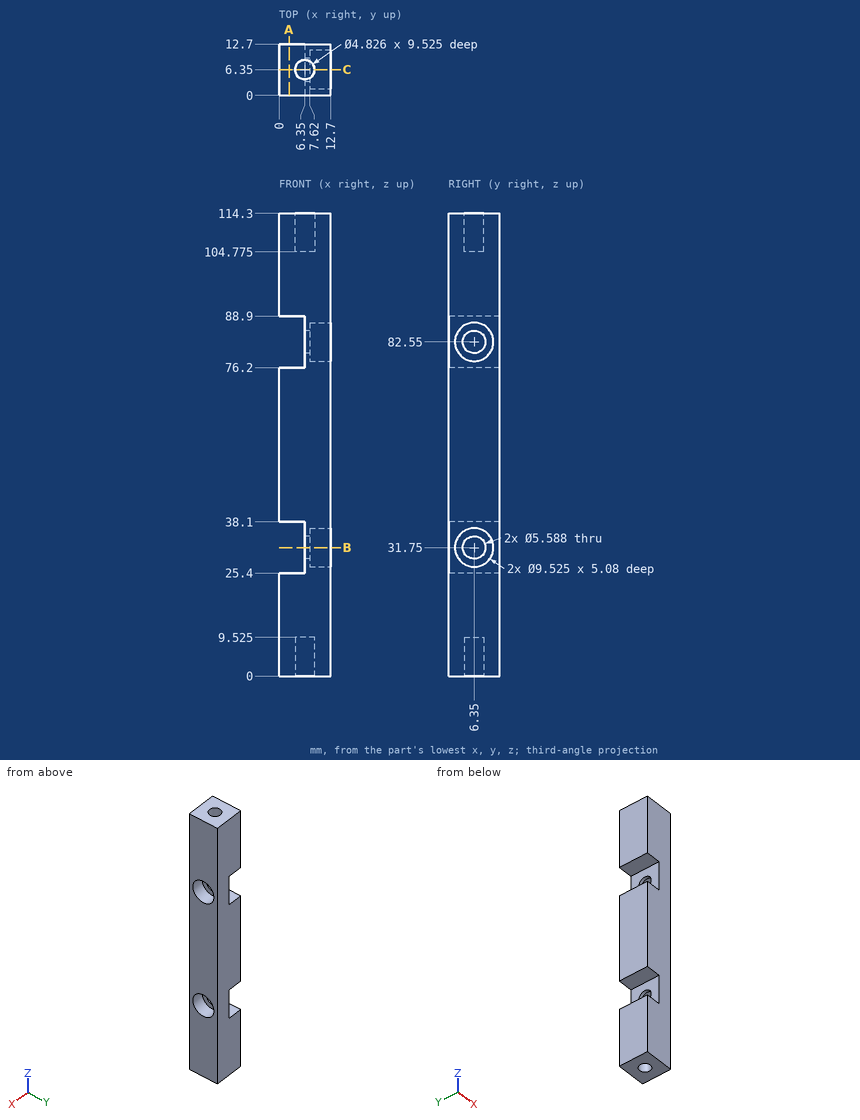
Here's the drawing with two shaded views (mm, measured from the low corner). I have some questions. Coordinates: 2 decimals unless noted, no trailing zeros. Write each loop counter-clockwise with the first axis right and the second up, starting at its lowest first coordinate (ties: lowest second). Pieces come first, ordered by that corner, then holes. Notation, with made-up numbers: (-34.5, 25.5) -> (-27.5, 25.5) arc R27 ccw to (-27.5, 45.5) -> close; hole circle Ø2 at (-29, 19). An arc over 180 degrees is marked (long way). Answer as CSV lines item,"result".
1) If we section it at A-A on x = 2.5: Please give me the cut outline in (y, z), then the cut area to 3 significant figures.
Check result:
outline,"(0, 0) -> (12.7, 0) -> (12.7, 25.4) -> (0, 25.4) -> close; (0, 38.1) -> (12.7, 38.1) -> (12.7, 76.2) -> (0, 76.2) -> close; (0, 88.9) -> (12.7, 88.9) -> (12.7, 114.3) -> (0, 114.3) -> close"
area,"1,130 mm²"
2) Will these pins go through, and if not, where does the flat tip stop? P1, Ø7.5, axis at y = 6.35, z = 31.75, coming from the +X side; P2, Ø3, axis at x = 6.35, y = 6.35, coming from the +Z side (3 decimals); P3, Ø3, axis at y = 10.5, z = 30.5, coming from the -X side.
Check result:
P1,"x = 7.62"
P2,"z = 104.775"
P3,"x = 6.35"
3) If we section it at C-C on y = 6.35: Count the separate pieces of the cut face and the enclosed holes in it, then the cut area to 3 significant figures.
Check result:
separate pieces,"3"
enclosed holes,"0"
area,"1,090 mm²"
4) If I drill on line 1 (Z direction, x = 6.25, y = 5) (3 decimals); line 2 (Z direction, x = 10.75, y = 2.5); line 3 (X direction, y = 6.35, z = 2.5), over which ranges is the centre line in solid material (lowest first)? Write a range as from..to.
Check result:
line 1,"9.525..25.4, 38.1..76.2, 88.9..104.775"
line 2,"0..28.95, 34.55..79.75, 85.35..114.3"
line 3,"0..3.94, 8.76..12.7"
5) If we section it at B-B on z = 31.75: Please give me the cut outline in (x, y).
Check result:
outline,"(6.35, 0) -> (12.7, 0) -> (12.7, 1.59) -> (7.62, 1.59) -> (7.62, 3.56) -> (6.35, 3.56) -> close; (6.35, 9.14) -> (7.62, 9.14) -> (7.62, 11.11) -> (12.7, 11.11) -> (12.7, 12.7) -> (6.35, 12.7) -> close"
